Source: CAD feature listing. Evaluate the final solid. Frame: model axes, mm. A direction names the side the tool comes from. Round coordinates to 2 decimals unless told otherwise and drop trailing zeros. Order: outer loops, then holes, each group sorted by start corner. A loop starts at its lowest first (then second) coordinate and runs counter-clockwise, first axis right, second up. Notation, with made-up numbers: (-11, -4.5) - (29, -4.5) arc R27 ccw to (29, 27.5) - close; hole circle Ø5 at (79, 38.25). An arc over 180 degrees is marked (long way). Put each result on its own line as item: value. Start each with the question number.
1) Contact query for flat-ended pins moving along their axis: P1, Ø6.5, axis at x = -24.5, z = -42.5, coming from the +Y side; P2, Ø10.5, axis at x = -25.5, z = 44.17, coming from the -Y side; P3, Ø5, axis at y = 5.5, z = -20.5, coming from the -X side; P4, Ø2, axis at x = 13.5, y = 27, coming from the -Z side. Output: stop coordinate, or through.
2) Mould query, pull axis Z, two halves, no side actions, for faces 4 (the face through (2.423, 16.358, -55.047)), 5 (the face through (48.95, 6.77, -0.46)), 6 (the face through (17.722, 17.008, 56.275)), 7 (the face through (-43, 0, 13)). Classes: +Z half, -Z half, draft (parallel to the pull), parting line (faces both ways), or undercut.
3) Section A-A on x = 0. State how many separate pieces and enclosed holes the cut face has, then the cut area to 3 significant figures.
4) Line query: probe 1 along X at (y, z) = (2.25, 0); probe 2 along X at (y, z) = (32, 0); probe 3 along Z at (x, y) = (-25, 6). Output: solid intervals per line, ascending. Write a range as [from, to].
5) Section B-B on z = -51. Output: boundary loops of the cut face in (x, y), then the cut area to 3 significant figures.
6) Section C-C on x = 25.5. Output: boundary loops of the cut face in (y, z).
7) Access query for faces 1 (the face through (40.262, 6.528, 24.633)), 2 (the face through (30.075, 4.31, -32.798)), 3 (the face through (-53, 5, -2)). Directions: +Z, -Z, +X, -X, +Y, -Y. A direction counts if a zero-diameter tool reaches every point of the face in a straight line with its end or side. Return the directions, or none.
```python
from build123d import *

# Parameters (mm, degrees)
SKETCH_1_R          = 59
EXTRUDE_1_DEPTH     = 34.5
SKETCH_2_R          = 57.6
CUT_EXTRUDE_1_DEPTH = 10.5
SKETCH_3_R          = 55.1
CUT_EXTRUDE_2_DEPTH = 15.5
SKETCH_4_R          = 44.5
CUT_EXTRUDE_3_DEPTH = 88.395652066
SKETCH_9_R          = 4
CUT_EXTRUDE_7_DEPTH = 4
SKETCH_10_R         = 2.1
CUT_EXTRUDE_8_DEPTH = 88.395652066
SKETCH_11_R         = 3.75
CUT_EXTRUDE_9_DEPTH = 5


with BuildPart() as part:
    # 草图1 → 凸台-拉伸1 (new body)
    with BuildSketch(Plane(origin=(0, 0, 0), x_dir=(1, 0, 0), z_dir=(0, 1, 0))):
        with Locations(Location((0, 0, 0), (0, 0, 270))):
            Circle(SKETCH_1_R)
    extrude(amount=EXTRUDE_1_DEPTH)

    # 草图2 → 切除-拉伸1 (cut)
    with BuildSketch(Plane(origin=(0, 34.5, 0), x_dir=(1, 0, 0), z_dir=(0, 1, 0))):
        with Locations(Location((0, 0, 0), (0, 0, 270))):
            Circle(SKETCH_2_R)
    extrude(amount=-CUT_EXTRUDE_1_DEPTH, mode=Mode.SUBTRACT)

    # 草图3 → 切除-拉伸2 (cut)
    with BuildSketch(Plane(origin=(0, 24, 0), x_dir=(1, 0, 0), z_dir=(0, 1, 0))):
        with Locations(Location((0, 0, 0), (0, 0, 270))):
            Circle(SKETCH_3_R)
    extrude(amount=-CUT_EXTRUDE_2_DEPTH, mode=Mode.SUBTRACT)

    # 草图4 → 切除-拉伸3 (cut, through all)
    with BuildSketch(Plane(origin=(0, 8.5, 0), x_dir=(1, 0, 0), z_dir=(0, 1, 0))):
        with Locations(Location((0, 0, 0), (0, 0, 270))):
            Circle(SKETCH_4_R)
    extrude(amount=-CUT_EXTRUDE_3_DEPTH, mode=Mode.SUBTRACT)

    # 草图9 → 切除-拉伸7 (cut)
    with BuildSketch(Plane(origin=(0, 8.5, 0), x_dir=(1, 0, 0), z_dir=(0, 1, 0))):
        with Locations(Location((-44.167295593, 25.5, 0), (0, 0, 270))):
            Circle(SKETCH_9_R)
        with Locations(Location((-25.5, 44.167295593, 0), (0, 0, 270))):
            Circle(SKETCH_9_R)
        with Locations(Location((25.5, 44.167295593, 0), (0, 0, 270))):
            Circle(SKETCH_9_R)
        with Locations(Location((44.167295593, 25.5, 0), (0, 0, 270))):
            Circle(SKETCH_9_R)
        with Locations(Location((44.167295593, -25.5, 0), (0, 0, 270))):
            Circle(SKETCH_9_R)
        with Locations(Location((25.5, -44.167295593, 0), (0, 0, 270))):
            Circle(SKETCH_9_R)
        with Locations(Location((-25.5, -44.167295593, 0), (0, 0, 270))):
            Circle(SKETCH_9_R)
        with Locations(Location((-44.167295593, -25.5, 0), (0, 0, 270))):
            Circle(SKETCH_9_R)
    extrude(amount=-CUT_EXTRUDE_7_DEPTH, mode=Mode.SUBTRACT)

    # 草图10 → 切除-拉伸8 (cut, through all)
    with BuildSketch(Plane(origin=(0, 8.5, 0), x_dir=(1, 0, 0), z_dir=(0, 1, 0))):
        with Locations(Location((0, 51, 0), (0, 0, 270))):
            Circle(SKETCH_10_R)
        with Locations(Location((51, 0, 0), (0, 0, 270))):
            Circle(SKETCH_10_R)
        with Locations(Location((0, -51, 0), (0, 0, 270))):
            Circle(SKETCH_10_R)
        with Locations(Location((-51, 0, 0), (0, 0, 270))):
            Circle(SKETCH_10_R)
    extrude(amount=-CUT_EXTRUDE_8_DEPTH, mode=Mode.SUBTRACT)

    # 草图11 → 切除-拉伸9 (cut)
    with BuildSketch(Plane.XZ):
        with Locations(Location((0, 51, 0), (0, 0, 270))):
            Circle(SKETCH_11_R)
        with Locations(Location((51, 0, 0), (0, 0, 270))):
            Circle(SKETCH_11_R)
        with Locations(Location((0, -51, 0), (0, 0, 270))):
            Circle(SKETCH_11_R)
        with Locations(Location((-51, 0, 0), (0, 0, 270))):
            Circle(SKETCH_11_R)
    extrude(amount=-CUT_EXTRUDE_9_DEPTH, mode=Mode.SUBTRACT)


solid = part.part
```
Answer sheet:
1. P1: y = 8.5
1. P2: y = 0
1. P3: x = -56.19
1. P4: z = -57.66
2. face 4: undercut
2. face 5: undercut
2. face 6: parting line
2. face 7: draft
3. separate pieces: 4
3. enclosed holes: 0
3. area: 292 mm^2
4. probe 1: [-59, -54.75], [-47.25, -44.5], [44.5, 47.25], [54.75, 59]
4. probe 2: [-59, -57.6], [57.6, 59]
4. probe 3: [-53.44, -48.14], [-40.2, -36.81], [36.81, 40.2], [48.14, 53.44]
5. outline: (-29.66, 0) - (-3.75, 0) - (-3.75, 5) - (-2.1, 5) - (-2.1, 8.5) - (-20.86, 8.5) - (-20.86, 24) - (-26.77, 24) - (-26.77, 34.5) - (-29.66, 34.5) - close; (2.1, 5) - (3.75, 5) - (3.75, 0) - (29.66, 0) - (29.66, 34.5) - (26.77, 34.5) - (26.77, 24) - (20.86, 24) - (20.86, 8.5) - (2.1, 8.5) - close
5. area: 786 mm^2
6. outline: (0, -53.2) - (34.5, -53.2) - (34.5, -51.65) - (24, -51.65) - (24, -48.84) - (8.5, -48.84) - (8.5, -48.17) - (4.5, -48.17) - (4.5, -40.17) - (8.5, -40.17) - (8.5, -36.47) - (0, -36.47) - close; (0, 36.47) - (8.5, 36.47) - (8.5, 40.17) - (4.5, 40.17) - (4.5, 48.17) - (8.5, 48.17) - (8.5, 48.84) - (24, 48.84) - (24, 51.65) - (34.5, 51.65) - (34.5, 53.2) - (0, 53.2) - close
7. face 1: +Y
7. face 2: +Y, -Y
7. face 3: -Y
